from build123d import *

# Parameters (mm, degrees)
SKETCH1_R           = 4.75
SKETCH1_R_2         = 3.25
BOSS_EXTRUDE1_DEPTH = 5
BOSS_EXTRUDE2_START = -2
BOSS_EXTRUDE2_DEPTH = 2
SKETCH3_R           = 1.025
CUT_EXTRUDE1_DEPTH  = 12.908505364
FILLET1_R           = 3.125
FILLET2_R           = 1
FILLET3_SIZE        = 3
FILLET3_SIZE_2      = 1


with BuildPart() as part:
    # Sketch1 → Boss-Extrude1 (new body)
    with BuildSketch(Plane(origin=(0, 0, 0), x_dir=(1, 0, 0), z_dir=(0, 1, 0))):
        with Locations(Location((0, 0, 0), (0, 0, 270))):
            Circle(SKETCH1_R)
        with Locations(Location((0, 0, 0), (0, 0, 270))):
            Circle(SKETCH1_R_2, mode=Mode.SUBTRACT)
    extrude(amount=BOSS_EXTRUDE1_DEPTH)

    # Sketch2 → Boss-Extrude2 (add)
    with BuildSketch(Plane(origin=(0, 5, 0), x_dir=(1, 0, 0), z_dir=(0, 1, 0)).offset(BOSS_EXTRUDE2_START)):
        with BuildLine():
            ThreePointArc((4.75, 0), (4.63829195, -1.024083876), (4.308421985, -2))
            Line((4.308421985, -2), (10.5, -2))
            Line((10.5, -2), (10.5, 2))
            Line((10.5, 2), (4.308421985, 2))
            ThreePointArc((4.308421985, 2), (4.63829195, 1.024083876), (4.75, 0))
        make_face()
        with BuildLine():
            Line((-10.5, -2), (-4.308421985, -2))
            ThreePointArc((-4.308421985, -2), (-4.75, 0), (-4.308421985, 2))
            Line((-4.308421985, 2), (-10.5, 2))
            Line((-10.5, 2), (-10.5, -2))
        make_face()
    extrude(amount=BOSS_EXTRUDE2_DEPTH)

    # Sketch3 → Cut-Extrude1 (cut, through all)
    with BuildSketch(Plane.XZ.offset(-3)):
        with Locations(Location((8.7, 0, 0), (0, 0, 270))):
            Circle(SKETCH3_R)
        with Locations(Location((-8.7, 0, 0), (0, 0, 270))):
            Circle(SKETCH3_R)
    extrude(amount=-CUT_EXTRUDE1_DEPTH, mode=Mode.SUBTRACT)

    # Fillet1
    fillet1_edges = [part.edges().sort_by_distance(p)[0] for p in [
        (4.308421985, 4, 2),
        (4.308421985, 4, -2),
        (-4.308421985, 4, -2),
        (-4.308421985, 4, 2),
    ]]
    fillet(fillet1_edges, radius=FILLET1_R)

    # Fillet2
    fillet2_edges = [part.edges().sort_by_distance(p)[0] for p in [
        (10.5, 4, 2),
        (10.5, 4, -2),
        (-10.5, 4, -2),
        (-10.5, 4, 2),
    ]]
    fillet(fillet2_edges, radius=FILLET2_R)

    # Fillet3
    # an asymmetric fillet: 3, 1 mm, written as the material it takes off along each edge
    with BuildSketch(Plane(origin=(0, 0, 0), x_dir=(0, 0, 1), z_dir=(-1, 0, 0))) as fillet3_piece_1:
        with BuildLine():
            Bezier((4.75, FILLET3_SIZE), (4.75, 0), (4.75 - FILLET3_SIZE_2, 0), weights=[1, 0.707106781, 1])
            Line((4.75 - FILLET3_SIZE_2, 0), (4.75, 0))
            Line((4.75, 0), (4.75, FILLET3_SIZE))
        make_face()
    revolve(axis=Axis((0, 0, 0), (0, 1, 0)), mode=Mode.SUBTRACT)


solid = part.part
The listing builds one solid part. Answer for the finished solid, in the listing's coordinates (mm). A direction names the side the tool comes from. Round coordinates to 2 decimals unless told otherwise and drop trailing zeros. Loops run counter-clockwise (first coordinate to the right, second up) from the corner with the lowest first, then second, coordinate; pieces in that order, holes last. Notation, with made-up numbers: M -13.75,16 L 30.25,16 A20 ccw 30.25,43 Z; hole C 65,-29 d7. An arc over 180 degrees is marked long. Write each question's results on one line, items separated by ' | '. Start each with the question number.
1) Straight lines are drawn through the part: probe 1 along X at (y, z) = (3.7, 0) (3 decimals); probe 2 along Z at (x, y) = (-2.25, 4); probe 3 along Y at (x, z) = (-5.5, 0). For each, find the intervals that lie inside material, in ascending order.
2) Find section A-A on x = -8.7. Write down the section's boundary in (y, z) (3 decimals), plus the area to 3 significant figures.
3) Which of the six approach directions +Z, -Z, +X, -X, +Y, -Y give full straight-line access (tool end or side, diameter ignored) to faces 4 (the flat face through (-8, 4, -2)), 5 (the flat face through (8, 4, 2)), 6 (the cylindrical face through (-10.199, 4.014, 1.715)), 7 (the flat face through (8, 4, -2)), 8 (the cylindrical face through (-7.684, 3.986, 0.133))?
4) Each of these flat-tipped pins is pushed along its axis until it touches: pin 1 (5 mm diameter, centred on x = 8.5, z = -0.5, fed in from -Y); pin 2 (1.8 mm diameter, centred on x = 8.7, z = 0, fed in from -Y); pin 3 (0.6 mm diameter, centred on x = 8.5, y = 4.5, fed in from +Z); pin 4 (1.6 mm diameter, centred on x = 8, y = 3.5, fed in from -Z). Where does it stop, or does it pass through?
5) Determine the mould class of faces 1 (the cylindrical face through (4.66, 4.01, 2.29)), 2 (the cylindrical face through (9.716, 3.986, 0.133)), 3 (the cylindrical face through (10.215, 4.014, -1.699)) for opening direction Z: pulls with the +Z half, pulls with the -Z half, needs draft (parallel to the pull), parting line crosses it, or undercut.
6) Find section C-C on x = 6.25. Write down the section's boundary in (y, z).
7) Find section B-B on y = 4.15. Write down the section's boundary in (x, z) (3 decimals), plus the area to 3 significant figures.
Final values:
1) probe 1: -10.5 to -9.725, -7.675 to -3.25, 3.25 to 7.675, 9.725 to 10.5 | probe 2: -4.18 to -2.35, 2.35 to 4.18 | probe 3: 3 to 5
2) outline: M 3,-2 L 5,-2 L 5,-1.025 L 3,-1.025 Z; M 3,1.025 L 5,1.025 L 5,2 L 3,2 Z | area: 3.90 mm²
3) face 4: -Z, -X, +Y, -Y | face 5: +Z, +X, +Y, -Y | face 6: +Z, -X, +Y, -Y | face 7: -Z, +X, +Y, -Y | face 8: +Y, -Y
4) pin 1: y = 3 | pin 2: through | pin 3: z = 2 | pin 4: z = -2
5) face 1: pulls with the +Z half | face 2: undercut | face 3: pulls with the -Z half
6) outline: M 3,-2 L 5,-2 L 5,2 L 3,2 Z
7) outline: M -10.5,-1 A1 ccw -9.5,-2 L -5.979,-2 A3.125 cw -3.606,-3.091 A4.75 ccw 3.606,-3.091 A3.125 cw 5.979,-2 L 9.5,-2 A1 ccw 10.5,-1 L 10.5,1 A1 ccw 9.5,2 L 5.979,2 A3.125 cw 3.606,3.091 A4.75 ccw -3.606,3.091 A3.125 cw -5.979,2 L -9.5,2 A1 ccw -10.5,1 Z; hole C -8.7,0 d2.05; hole C 0,0 d6.5; hole C 8.7,0 d2.05 | area: 78.9 mm²
